Can you work these out from the model? Positions are in its coordinate system, mm. A direction names the side the tool comes from. Coordinates: 2 decimals unless noted, no trailing zeros. Write each loop counter-clockwise with the first axis right and the second up, starting at its lowest first coordinate (ties: lowest second). Pieces come first, ordered by that corner, then holes. Notation, with made-up numbers: (59, 20.5) -> (68, 20.5) arc R20 ccw to (68, 27.5) -> close; hole circle Ø10 at (81, -33). An arc over 180 degrees is marked (long way). Answer as CSV lines item,"result". Start each with the question number.
```python
from build123d import *

# Parameters (mm, degrees)
ESQUISSE1_R          = 3.5
BOSS_EXTRU_1_DEPTH   = 200
BOSS_EXTRU_1_2_DEPTH = 200
ESQUISSE2_W          = 70
ESQUISSE2_H          = 12
BOSS_EXTRU_2_DEPTH   = 10
ESQUISSE3_W          = 70
ESQUISSE3_H          = 12
BOSS_EXTRU_3_DEPTH   = 10


with BuildPart() as part:
    # Esquisse1 → Boss.-Extru.1 (new body)
    with BuildSketch(Plane.XY):
        with Locations((-15.470635051, 10.736898533)):
            Circle(ESQUISSE1_R)
    extrude(amount=BOSS_EXTRU_1_DEPTH)



with BuildPart() as body_2:
    # Esquisse1 → Boss.-Extru.1 2 (new body)
    with BuildSketch(Plane.XY):
        with Locations((9.529364949, 10.736898533)):
            Circle(ESQUISSE1_R)
    extrude(amount=BOSS_EXTRU_1_2_DEPTH)


with BuildPart() as part_1:
    add(part.part)

    add(body_2.part)  # Boss.-Extru.2 merges body 2
    # Esquisse2 → Boss.-Extru.2 (add)
    with BuildSketch(Plane(origin=(0, 0, 0), x_dir=(-1, 0, 0), z_dir=(0, 0, -1))):
        with Locations((2.970635051, 10.736898533)):
            Rectangle(ESQUISSE2_W, ESQUISSE2_H)
    extrude(amount=BOSS_EXTRU_2_DEPTH)

    # Esquisse3 → Boss.-Extru.3 (add)
    with BuildSketch(Plane.XY.offset(200)):
        with Locations((-2.970635051, 10.736898533)):
            Rectangle(ESQUISSE3_W, ESQUISSE3_H)
    extrude(amount=BOSS_EXTRU_3_DEPTH)


solid = part_1.part
```
Q1. Imagine slicing it at C-C (z = 40). Write out the boundary of the cut face in (x, y).
Q2. I need wall thicknesses on L1, parallel to Z at x = -10, y = 10.5; L2, parallel to X at y = 9.75, z = 140.5; L3, parallel to X at y = 9.25, z = 165.5. Which ranges of each line are inside material? Lowest first, please.
Q3. Imagine slicing it at B-B (x = -17). Write out the boundary of the cut face in (y, z), then the cut area to 3 significant figures.
Q4. If we mould it in two halves opening along Z, with no side actions, what happens to faces 3 (the face through (-2, 11, 0)), 4 (the face through (-2, 11, -10)), 5 (the face through (-3, 11, 210))? For each: released by +Z, released by -Z, zero draft, split by the parting line, or undercut.
Q5. Which directions (+Z, -Z, +X, -X, +Y, -Y) give clear straight access to the entire face, cutting with the end or side of a thin tool? Please do faces 1 (the face through (-3, 4.737, 205)), 2 (the face through (-15.926, 14.207, 98.6)).
Q6. Imagine slicing it at A-A (x = 16.5). Write out the boundary of the cut face in (y, z), then the cut area to 3 significant figures.
Q7. For pin 1 (6 mm diameter, centred on x = 8, z = 96, fed in from -Y); pin 2 (1.5 mm diameter, centred on x = 12, z = 79.5, fed in from -Y); pin 3 (6 mm diameter, centred on y = 9.5, z = 38.5, fed in from -X), each with a flat end and sliding along its axis, tell me the tip position at first contact or that it passes through.
Entries:
1,outline,"circle Ø7 at (-15.47, 10.74); circle Ø7 at (9.53, 10.74)"
2,L1,"-10 to 0, 200 to 210"
2,L2,"-18.83 to -12.11, 6.17 to 12.89"
2,L3,"-18.64 to -12.3, 6.36 to 12.7"
3,outline,"(4.74, -10) -> (16.74, -10) -> (16.74, 0) -> (13.89, 0) -> (13.89, 200) -> (16.74, 200) -> (16.74, 210) -> (4.74, 210) -> (4.74, 200) -> (7.59, 200) -> (7.59, 0) -> (4.74, 0) -> close"
3,area,"1,500 mm2"
4,face 3,"undercut"
4,face 4,"released by -Z"
4,face 5,"released by +Z"
5,face 1,"+Z, -Z, +X, -X, -Y"
5,face 2,"none"
6,outline,"(4.74, -10) -> (16.74, -10) -> (16.74, 0) -> (4.74, 0) -> close; (4.74, 200) -> (16.74, 200) -> (16.74, 210) -> (4.74, 210) -> close"
6,area,"240 mm2"
7,pin 1,"y = 7.24"
7,pin 2,"y = 7.69"
7,pin 3,"x = -18.97"
